For this review, take the finished solid that the model builds, in its own axes (mm). Face numbers are marked on the shaded views. A direction names the side the tool comes from. Give positions to 0.01 mm unless a question says otherwise; leave off trailing zeros. Write each loop counter-clockwise with the first axis right and the second up, starting at its lowest first coordinate (ties: lowest second). Pieces come first, ordered by that corner, then holes. Notation, with made-up numbers: M 1.25,64 L 11.25,64 A19 cw 11.25,83 Z; hole C 3,-1 d2. An arc over 180 degrees is marked long. Answer as a JSON object with one key per item and string values. Group by question number.
```python
from build123d import *

# Parameters (mm, degrees)
CROQUIS2_R                   = 3.5
SALIENTE_EXTRUIR1_DEPTH      = 27
ROSCA1_PITCH                 = 1
CROQUIS5_R                   = 12.45
CROQUIS5_R_2                 = 2.45
CORTAR_EXTRUIR_L_MINA1_DEPTH = 2.1
CROQUIS6_R                   = 1.2
CORTAR_EXTRUIR1_DEPTH        = 28.449954628
CHAFL_N1_SIZE                = 1
CROQUIS8_R                   = 1.5875
CORTAR_EXTRUIR2_DEPTH        = 5
CHAFL_N2_SIZE                = 1


with BuildPart() as part:
    # Croquis2 → Saliente-Extruir1 (new body)
    with BuildSketch(Plane(origin=(0, 0, 0), x_dir=(1, 0, 0), z_dir=(0, 1, 0))):
        with Locations(Location((0, 0, 0), (0, 0, 270))):
            Circle(CROQUIS2_R)
    extrude(amount=SALIENTE_EXTRUIR1_DEPTH)

    # Rosca1: the profile of Perfil de rosca1 profile screwed along a right-hand helix of 6 turns, 8 arcs to a turn; built about Z, then put on its axis
    rosca1_z = Axis((0, 0, 0), (0, 0, 1))
    rosca1_corners = [(3.5003, 0, -0.000173205), (3.5003, 0, 0.875173202), (2.958734125, 0, 0.562499999), (2.958734125, 0, 0.312499999)]
    with BuildLine(mode=Mode.PRIVATE) as rosca1_profile:
        Line(rosca1_corners[0], rosca1_corners[1])
        Line(rosca1_corners[1], rosca1_corners[2])
        Line(rosca1_corners[2], rosca1_corners[3])
        Line(rosca1_corners[3], rosca1_corners[0])
    rosca1_cap = Face(rosca1_profile.wire())
    rosca1_turn_angles = [0, 22.5, 45, 67.5, 90, 112.5, 135, 157.5, 180, 202.5, 225, 247.5, 270, 292.5, 315, 337.5, 360]
    rosca1_turn_weights = [1, 0.9238795325112867, 1, 0.9238795325112867, 1, 0.9238795325112867, 1, 0.9238795325112867, 1, 0.9238795325112867, 1, 0.9238795325112867, 1, 0.9238795325112867, 1, 0.9238795325112867, 1]
    rosca1_turn_rails = [Edge.make_bspline([Vector(p[0], p[1], 0).rotate(rosca1_z, rosca1_turn_angles[k]) / rosca1_turn_weights[k] + Vector(0, 0, p[2] + ROSCA1_PITCH * rosca1_turn_angles[k] / 360) for k in range(17)], [0, 0, 0, 1, 1, 2, 2, 3, 3, 4, 4, 5, 5, 6, 6, 7, 7, 8, 8, 8], 2, rosca1_turn_weights) for p in rosca1_corners]
    rosca1_turn_sides = [Face.make_surface_from_curves(rosca1_turn_rails[p[0]], rosca1_turn_rails[p[1]]) for p in [(0, 1), (1, 2), (2, 3), (3, 0)]]
    rosca1 = Plane(origin=(0, -1, 0), x_dir=(1, 0, 0), z_dir=(0, 1, 0)) * Solid(Shell([*[p.moved(Location((0, 0, ROSCA1_PITCH * i))) for i in range(6) for p in rosca1_turn_sides], rosca1_cap, rosca1_cap.rotate(rosca1_z, 2160).moved(Location((0, 0, ROSCA1_PITCH * 2160 / 360)))]))
    add(rosca1, mode=Mode.SUBTRACT)

    # Croquis5 → Cortar-Extruir-Lámina1 (cut)
    with BuildSketch(Plane(origin=(0, 5, 0), x_dir=(-1, 0, 0), z_dir=(0, -1, 0))):
        Circle(CROQUIS5_R)
        Circle(CROQUIS5_R_2, mode=Mode.SUBTRACT)
    extrude(amount=-CORTAR_EXTRUIR_L_MINA1_DEPTH, mode=Mode.SUBTRACT)

    # Croquis6 → Cortar-Extruir1 (cut, through all)
    with BuildSketch(Plane(origin=(0, 27, 0), x_dir=(1, 0, 0), z_dir=(0, 1, 0))):
        with Locations(Location((0, 0, 0), (0, 0, 270))):
            Circle(CROQUIS6_R)
    extrude(amount=-CORTAR_EXTRUIR1_DEPTH, mode=Mode.SUBTRACT)

    # Chaflán1
    chafl_n1_edges = [part.edges().sort_by_distance(p)[0] for p in [
        (0, 7.1, -3.5),
    ]]
    chamfer(chafl_n1_edges, length=CHAFL_N1_SIZE)

    # Croquis8 → Cortar-Extruir2 (cut)
    with BuildSketch(Plane(origin=(0, 27, 0), x_dir=(1, 0, 0), z_dir=(0, 1, 0))):
        with Locations(Location((0, 0, 0), (0, 0, 270))):
            Circle(CROQUIS8_R)
    extrude(amount=-CORTAR_EXTRUIR2_DEPTH, mode=Mode.SUBTRACT)

    # Chaflán2
    # the kernel refuses this chamfer: 1 mm, written as the material it takes off along each edge
    with BuildSketch(Plane(origin=(0, 22, 0), x_dir=(0, 0, 1), z_dir=(-1, 0, 0))) as chafl_n2_piece_1_section:
        Polygon((1.2 + CHAFL_N2_SIZE, 0), (1.2, -CHAFL_N2_SIZE), (1.2, 0), align=None)
    chafl_n2_piece_1 = revolve(axis=Axis((0, 22, 0), (0, 1, 0)), mode=Mode.PRIVATE)
    chafl_n2_piece_1 = chafl_n2_piece_1 & Plane(origin=(0, 21.189751439, 0), x_dir=(0, 0, 1), z_dir=(0, 1, 0)) * Cylinder(1.5875, 9, mode=Mode.PRIVATE)
    add(chafl_n2_piece_1, mode=Mode.SUBTRACT)


solid = part.part
```
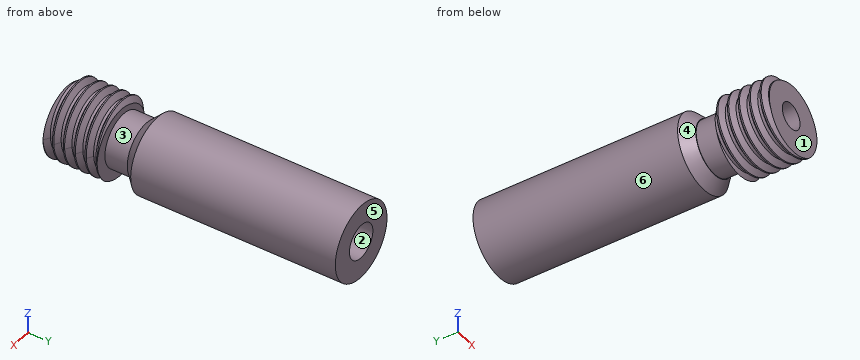
Item 1: Consider section A-A (y = 6.25). Give the boundary of the cut face in (x, z).
Item 2: Draft analysis for pull direction Y (two halves, no side actions). For the marked faces 3, 4, 5 and 6, state which applies: released by +Y, released by -Y, zero draft, split by the parting line, or undercut.
Item 3: To check wall thickness, follow probe 1 along X at (y, z) = (9.75, 0); probe 2 along Y at (x, z) = (-2, 1.75); probe 3 along Y at (x, z) = (-3, 1). State the ranges of each line that lie inside material, in increasing order.
Item 4: Machinability: for the marked faces 1 and 2, which of the approach directions +Z, -Z, +X, -X, +Y, -Y give a long, thin tool a straight path to every point of the face, cutting with its end or side? Answer none if there is none.
Item 5: Consider section B-B (y = 11). Give the boundary of the cut face in (x, z).
Item 6: Insertion check: P1, Ø1.5, axis at y = 22, z = -1, coming from the +X side; P2, Ø1.5, axis at y = 23.5, z = 1.5, coming from the +X side; P3, Ø3, axis at x = 0, z = 0, coming from the +Y side. Each pin has a flat end and moves straight along its axis. Give the tip position at first contact, or say it passes through.
Result set:
{
 "1": {"outline": "C 0,0 d4.9; hole C 0,0 d2.4"},
 "2": {"face 3": "undercut", "face 4": "undercut", "face 5": "released by +Y", "face 6": "zero draft"},
 "3": {"probe 1": "x = -3.5 to -1.2, 1.2 to 3.5", "probe 2": "y = 0 to 5, 7.26 to 27", "probe 3": "y = 0.23 to 0.75, 1.23 to 1.75, 2.23 to 2.75, 3.23 to 3.75, 4.23 to 4.75, 7.76 to 27"},
 "4": {"face 1": "+Z, -Z, +X, -X, -Y", "face 2": "+Y"},
 "5": {"outline": "C 0,0 d7; hole C 0,0 d2.4"},
 "6": {"P1": "stops at x = 3.49", "P2": "stops at x = 3.42", "P3": "stops at y = 21.3"}
}
